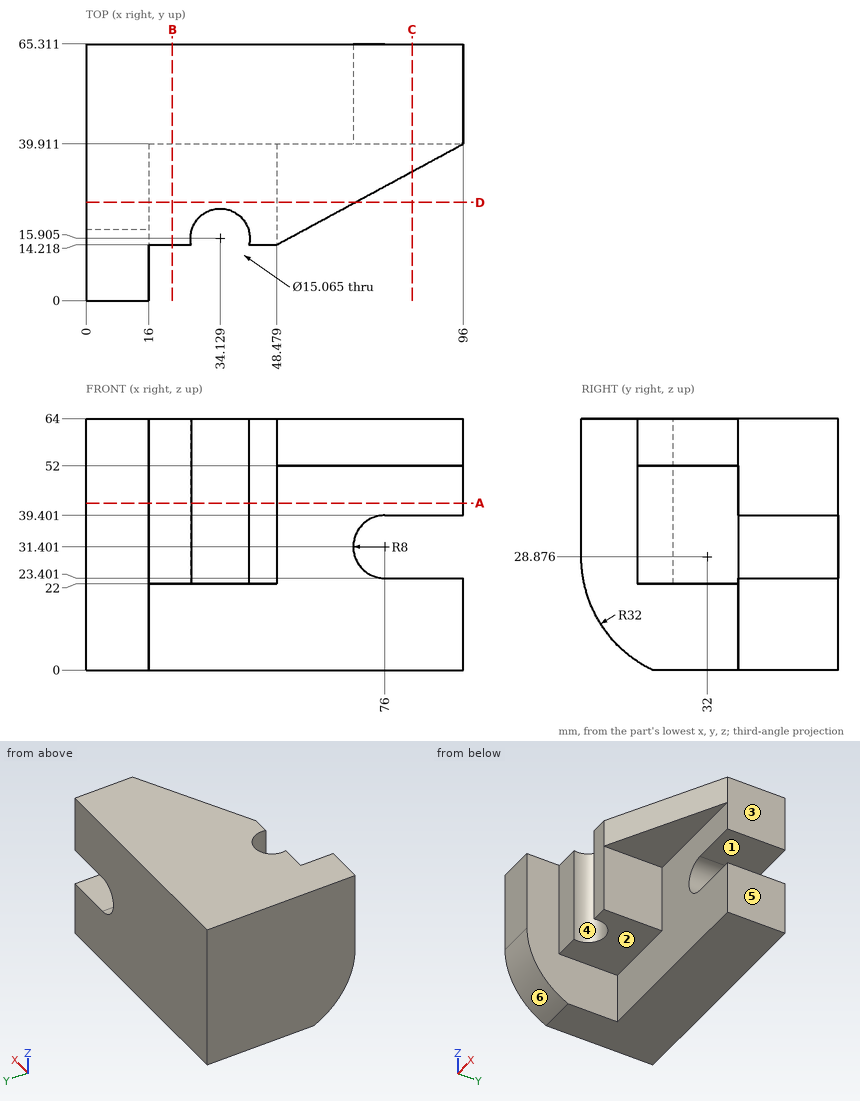
Verification items for this drawing (mm, ordinates from the low corner). A direction names the side the tool comes from. Give positions to 0.01 mm unless a question says otherwise; leave off trailing zeros. Write each loop counter-clockwise with the first axis right and the second up, starting at its lowest first coordinate (ties: lowest second). Pieces come first, ordered by that corner, then holes. Notation, with made-up numbers: (19.25, -1.75) -> (40.25, -1.75) arc R21 ccw to (40.25, 34.25) -> close; hole circle Ø8 at (-11, 3.25). An arc over 180 degrees is marked (long way). Use CSV: the item, a comma, the result in double quotes.
(1) Sectioned sample at A-A (z = 42.5). Record the cut outline in (x, y) (1 decimal), plus the area to 3 significant figures.
Derived:
outline,"(0, 0) -> (16, 0) -> (16, 14.2) -> (26.8, 14.2) arc R7.5 cw (long way) to (41.5, 14.2) -> (48.5, 14.2) -> (48.5, 39.9) -> (96, 39.9) -> (96, 65.3) -> (0, 65.3) -> close"
area,"3,800 mm^2"
(2) Release check for a two-part mould opening along X. For the marked faces 4, 5 and 6 record: +X half, -X half, draft (parallel to the pull), parting line (faces both ways), or undercut.
Derived:
face 4,"undercut"
face 5,"+X half"
face 6,"draft"
(3) Sectioned sample at D-D (y = 25). Record the cut outline in (x, z), plus the area to 3 significant figures.
Derived:
outline,"(0, 0) -> (16, 0) -> (16, 22) -> (48.48, 22) -> (48.48, 52) -> (68.42, 52) -> (68.42, 64) -> (0, 64) -> close"
area,"2,630 mm^2"
(4) Sectioned sample at C-C (x = 83). Record the cut outline in (y, z).
Derived:
outline,"(32.88, 52) -> (39.91, 52) -> (39.91, 39.4) -> (65.31, 39.4) -> (65.31, 64) -> (32.88, 64) -> close; (39.91, 0) -> (65.31, 0) -> (65.31, 23.4) -> (39.91, 23.4) -> close"
(5) Go/stop test with flat-tipped pins: pin 1 (13 mm diameter, centred on x = 26, y = 29, fed in from -Z); pin 2 (20.5 mm diameter, centred on y = 28.5, z = 32.5, fed in from +X); pin 3 (2 mm diameter, centred on y = 25, z = 8, fed in from +X). Record where each tip stops, or that it passes through.
Derived:
pin 1,"stops at z = 22"
pin 2,"stops at x = 48.48"
pin 3,"stops at x = 16"
(6) Material ranges on L1, parallel to Z at x = 27, y = 36; L2, parallel to X at y = 12.5, z = 57; L3, parallel to Y at x = 18, z = 32.5, recorded low to high.
Derived:
L1,"z = 22 to 64"
L2,"x = 0 to 16"
L3,"y = 14.22 to 65.31"
(7) Set-up check for the marked faces 1, 2 and 3: record each of +Z, -Z, +X, -X, +Y, -Y from which the full face is reachable in a straight line by a thin tool's end or side.
Derived:
face 1,"+X, +Y, -Y"
face 2,"-Z, +X, -Y"
face 3,"+Z, -Z, +X, +Y, -Y"
(8) Sectioned sample at B-B (x = 22). Record the cut outline in (y, z).
Derived:
outline,"(14.22, 22) -> (39.91, 22) -> (39.91, 0) -> (65.31, 0) -> (65.31, 64) -> (14.22, 64) -> close"
